Autodesk Inventor part; units mm, degrees
ref_plane "YZ Plane" through (0, 0, 0) normal (1, 0, 0) x (0, 1, 0)
ref_plane "XZ Plane" through (0, 0, 0) normal (0, 1, 0) x (-1, 0, 0)
ref_plane "XY Plane" through (0, 0, 0) normal (0, 0, 1) x (1, 0, 0)
sketch "Sketch1" plane through (0, 0, 0) normal (0, 0, 1) x (1, 0, 0)
  line L0 (0, 0) -> (0, -2.3114)
  line L1 (0, 0) -> (0, 2.3114)
  line L2 (0, 0) -> (2.3114, 0)
  line L3 (0, 0) -> (-2.3114, 0)
  line L4 (0, -2.3114) -> (-1.8034, -2.3114)
  line L5 (-2.3114, -1.8034) -> (-2.3114, 1.8034)
  line L6 (-1.8034, 2.3114) -> (1.8034, 2.3114)
  line L7 (2.3114, 1.8034) -> (2.3114, -1.8034)
  line L8 (1.8034, -2.3114) -> (0, -2.3114)
  arc A0 (1.8034, -2.3114) -> (2.3114, -1.8034) centre (1.8034, -1.8034) ccw
  arc A1 (-2.3114, -1.8034) -> (-1.8034, -2.3114) centre (-1.8034, -1.8034) ccw
  arc A2 (-1.8034, 2.3114) -> (-2.3114, 1.8034) centre (-1.8034, 1.8034) ccw
  arc A3 (2.3114, 1.8034) -> (1.8034, 2.3114) centre (1.8034, 1.8034) ccw
  circle A4 centre (6.2738, -6.35) radius 2.1844
  circle A5 centre (6.2738, 6.35) radius 2.1844
  line L9 (-6.4262, -10.16) -> (-6.4262, -8.5344)
  line L10 (-6.4262, -2.54) -> (-6.4262, -4.1656)
  arc A6 (-6.4262, -8.5344) -> (-6.4262, -4.1656) centre (-6.4262, -6.35) ccw
  arc A7 (-6.4262, 4.1656) -> (-6.4262, 8.5344) centre (-6.4262, 6.35) ccw
  line L11 (-6.4262, 2.54) -> (-6.4262, 4.1656)
  line L12 (-6.4262, 8.5344) -> (-6.4262, 10.16)
  circle A8 centre (0, -12.7) radius 2.1971
  circle A9 centre (0, 12.7) radius 2.1971
  line L13 (-3.122, 14.8838) -> (-6.4262, 10.16)
  line L14 (-6.4262, -10.16) -> (-3.122, -14.8838)
  line L15 (8.9841, -9.0278) -> (2.7103, -15.3778)
  line L16 (10.0838, -6.35) -> (10.0838, 6.35)
  line L17 (8.9841, 9.0278) -> (2.7103, 15.3778)
  arc A10 (-3.122, -14.8838) -> (2.7103, -15.3778) centre (0, -12.7) ccw
  arc A11 (8.9841, -9.0278) -> (10.0838, -6.35) centre (6.2738, -6.35) ccw
  arc A12 (10.0838, 6.35) -> (8.9841, 9.0278) centre (6.2738, 6.35) ccw
  arc A13 (2.7103, 15.3778) -> (-3.122, 14.8838) centre (0, 12.7) ccw
  line L18 (-6.4262, 2.54) -> (-6.4262, -2.54)
  point P0 (2.3114, -2.3114)
  dimension "d0" = 2.3114
  dimension "d1" = 2.3114
  dimension "d2" = 2.3114
  dimension "d3" = 2.3114
  dimension "d4" = 0.508
extrude "Extrusion1" add sketch "Sketch1" along normal blind 1.524
properties part number "pto-shaft-support"
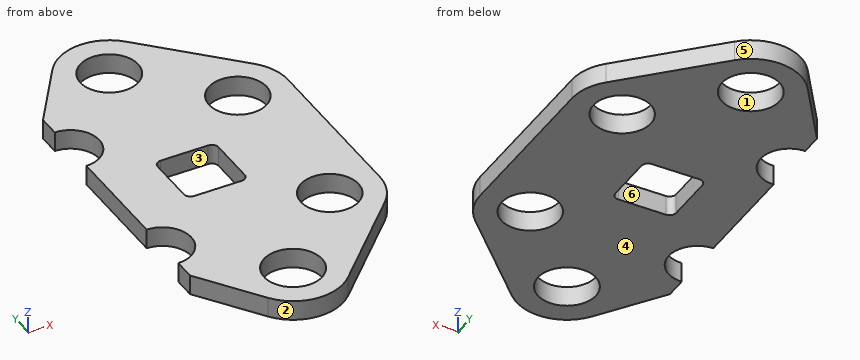
Design review of the part built by this model. Coordinates are the model's own, in mm. Face numbers are marked on the shaded views. A direction names the side the tool comes from. Round coordinates to 2 decimals unless told otherwise and drop trailing zeros. Loops run counter-clockwise (first coordinate to the right, second up) from the corner with the lowest first, then second, coordinate; pieces in that order, holes last. Notation, with made-up numbers: M 24.25,48 L 75.25,48 A11 ccw 75.25,60 Z; hole C -16,14 d1. An arc over 180 degrees is marked long. Answer as a JSON object with one key per item and string values.
Item 1: We need section B-B on z = 0.8. Give the boundary of the cut face in (x, y).
Answer sheet:
{"outline": "M -6.43,-10.16 L -3.12,-14.88 A3.81 ccw 2.71,-15.38 L 8.98,-9.03 A3.81 ccw 10.08,-6.35 L 10.08,6.35 A3.81 ccw 8.98,9.03 L 2.71,15.38 A3.81 ccw -3.12,14.88 L -6.43,10.16 L -6.43,8.53 A2.18 cw -6.43,4.17 L -6.43,-4.17 A2.18 cw -6.43,-8.53 Z; hole M -2.31,-1.8 A0.51 ccw -1.8,-2.31 L 1.8,-2.31 A0.51 ccw 2.31,-1.8 L 2.31,1.8 A0.51 ccw 1.8,2.31 L -1.8,2.31 A0.51 ccw -2.31,1.8 Z; hole C 0,-12.7 d4.39; hole C 0,12.7 d4.39; hole C 6.27,-6.35 d4.37; hole C 6.27,6.35 d4.37"}
Item 2: Machinability: for the marked faces 5 and 6, which of the approach directions +Z, -Z, +X, -X, +Y, -Y give a long, thin tool a straight path to every point of the face, cutting with its end or side? Answer none if there is none.
Answer sheet:
{"face 5": "+Z, -Z, +Y", "face 6": "+Z, -Z"}
Item 3: Wall thickness on L1, parallel to Y at x = -5.25, z = 1.4; L2, parallel to Y at x = -2, z = 0.3; L3, parallel to Y at x = 0.75, z = 1.05: over which ranges is each line inside the solid? List them lowest first. Write a range as from..to.
Answer sheet:
{"L1": "y = -11.84..-8.19, -4.51..4.51, 8.19..11.84", "L2": "y = -15.94..-13.61, -11.79..-2.27, 2.27..11.79, 13.61..15.94", "L3": "y = -16.44..-14.77, -10.63..-2.31, 2.31..10.63, 14.77..16.44"}
Item 4: We need section D-D on x = 6.25. Give the boundary of the cut face in (y, z), and give its area (3 significant figures).
Answer sheet:
{"outline": "M -11.8,0 L -8.53,0 L -8.53,1.52 L -11.8,1.52 Z; M -4.17,0 L 4.17,0 L 4.17,1.52 L -4.17,1.52 Z; M 8.53,0 L 11.8,0 L 11.8,1.52 L 8.53,1.52 Z", "area": "22.6 mm^2"}
Item 5: The part is to be moulded in two halves that separate along X. For the marked faces 1, 2, 3 and 4, say which applies: pulls with the +X half, pulls with the -X half, needs draft (parallel to the pull), parting line crosses it, or undercut.
Answer sheet:
{"face 1": "undercut", "face 2": "parting line crosses it", "face 3": "undercut", "face 4": "needs draft"}
Item 6: We need section C-C on y = 12. Give the boundary of the cut face in (x, z).
Answer sheet:
{"outline": "M -5.14,0 L -2.08,0 L -2.08,1.52 L -5.14,1.52 Z; M 2.08,0 L 6.05,0 L 6.05,1.52 L 2.08,1.52 Z"}
Item 7: We need section A-A on x = 0. Give the boundary of the cut face in (y, z), and give its area (3 significant figures).
Answer sheet:
{"outline": "M -16.51,0 L -14.9,0 L -14.9,1.52 L -16.51,1.52 Z; M -10.5,0 L -2.31,0 L -2.31,1.52 L -10.5,1.52 Z; M 2.31,0 L 10.5,0 L 10.5,1.52 L 2.31,1.52 Z; M 14.9,0 L 16.51,0 L 16.51,1.52 L 14.9,1.52 Z", "area": "29.9 mm^2"}
